Verification items for the finished model (mm, model axes). A direction names the side the tool comes from. Give positions to 0.01 mm unless a question says otherwise; leave off trailing zeros. Loops run counter-clockwise (first coordinate to the right, second up) from the corner with the lowest first, then second, coordinate; pieces in that order, holes last. Notation, with made-up numbers: (69, 28) - (127, 28) arc R32 ccw to (127, 67) - close; hole circle Ø7 at (6, -39). An arc over 180 degrees is marked (long way). One line per question, with ' | ' between items. Start each with the question number.
1. Mould release check, pull along X, two halves, no side actions. Record for faces 5 (the face through (54.27, 10.17, -9.33)), 6 (the face through (6.944, 10.666, -7.841)), 7 (the face through (89.5, 0, 0)): +X half, -X half, draft (parallel to the pull), parting line (faces both ways), or undercut.
2. Depth check by flat-ended pin: pin 1 Ø12 at (y, z) = (-2.5, 8) entering from -X; pin 2 Ø2.5 at (y, z) = (-9.19, -9.19) entering from -X; pin 3 Ø2 at (x, y) = (77.5, -6) entering from -Z; pin 4 Ø4 at (x, z) = (36.5, -2) entering from +Y. Enter the tip coordinate at first touch or a pass-through.
3. Thickness scan on line 1 along X through (y, z) = (6.5, 13); line 2 along Z through (x, y) = (10, 10); line 3 along X through (y, z) = (6.5, 11.5). Record the ranges inside material, lowest first. Write a range as from..to.
4. Tool access check on faces 1 (the face through (2, -9, 0)), 2 (the face through (2, 9, 0)), 3 (the face through (11, 9, -9)), 4 (the face through (73, -4.8, -13.1)). Record the directions out of +Z, -Z, +X, -X, +Y, -Y that give a thin tool (end or side, any length) a straight path to the whole face; none if there is none.
5. Section check C-C, the plane x = 44. Enter the section's corners in (y, z), then the cut area to 3 significant figures.
6. Section check A-A, the plane z = 0. Enter the section's corners in (x, y).
7. Section check B-B, the plane y = 0. Enter the section's corners in (x, z).
8. Section check D-D, the plane x = 26. Enter the section's corners in (y, z).
from build123d import *

# Parameters (mm, degrees)
SKETCH2_W           = 16.5
SKETCH2_H           = 16
SKETCH4_R           = 2
CUT_EXTRUDE1_DEPTH  = 8
SKETCH5_R           = 3
BOSS_EXTRUDE1_DEPTH = 16
CUT_EXTRUDE2_START  = -3
CUT_EXTRUDE2_DEPTH  = 3


with BuildPart() as part:
    # Sketch1 → Revolve1 (revolve)
    with BuildSketch(Plane.XY, mode=Mode.PRIVATE) as revolve1_sk:
        Polygon((0, 0), (0, 10), (3, 10), (3, 16), (35, 16), (35, 13.8), (73, 13.8), (73, 0), align=None)
    revolve(revolve1_sk.sketch.rotate(Axis((0, 0, 0), (1, 0, 0)), 180), axis=Axis((0, 0, 0), (1, 0, 0)))

    # Sketch2 → Revolve2 (revolve)
    with BuildSketch(Plane.XY, mode=Mode.PRIVATE) as revolve2_sk:
        with Locations((81.25, 8)):
            Rectangle(SKETCH2_W, SKETCH2_H)
    revolve(revolve2_sk.sketch.rotate(Axis((73, 0, 0), (1, 0, 0)), 180), axis=Axis((73, 0, 0), (1, 0, 0)))

    # Sketch4 → Cut-Extrude1 (cut)
    with BuildSketch(Plane.ZY.offset(-3)):
        with Locations(Location((9.192388155, 9.192388155, 0), (0, 0, 270))):
            Circle(SKETCH4_R)
        with Locations(Location((9.192388155, -9.192388155, 0), (0, 0, 270))):
            Circle(SKETCH4_R)
        with Locations(Location((-9.192388155, -9.192388155, 0), (0, 0, 270))):
            Circle(SKETCH4_R)
        with Locations(Location((-9.192388155, 9.192388155, 0), (0, 0, 270))):
            Circle(SKETCH4_R)
    extrude(amount=-CUT_EXTRUDE1_DEPTH, mode=Mode.SUBTRACT)

    # Sketch5 → Boss-Extrude1 (add)
    with BuildSketch(Plane.ZY):
        with Locations(Location((0, 0, 0), (0, 0, 270))):
            Circle(SKETCH5_R)
    extrude(amount=BOSS_EXTRUDE1_DEPTH)

    # Sketch6 → Cut-Extrude2 (cut)
    with BuildSketch(Plane.ZY.offset(CUT_EXTRUDE2_START)):
        with BuildLine():
            Line((4.358898944, -9), (-4.358898944, -9))
            ThreePointArc((-4.358898944, -9), (0, -10), (4.358898944, -9))
        make_face()
        with BuildLine():
            ThreePointArc((4.358898944, 9), (0, 10), (-4.358898944, 9))
            Line((-4.358898944, 9), (4.358898944, 9))
        make_face()
    extrude(amount=CUT_EXTRUDE2_DEPTH, mode=Mode.SUBTRACT)


solid = part.part
Results list:
1) face 5: undercut | face 6: draft | face 7: +X half
2) pin 1: x = -16 | pin 2: x = 11 | pin 3: z = -15.2 | pin 4: y = 15.99
3) line 1: 3..35, 73..89.5 | line 2: -12.49..-11.02, -7.36..7.36, 11.02..12.49 | line 3: 3..89.5
4) face 1: +Z, -Z, -X, -Y | face 2: +Z, -Z, -X, +Y | face 3: -X | face 4: none
5) outline: circle Ø27.6 at (0, 0) | area: 598 mm²
6) outline: (-16, -3) - (0, -3) - (0, -9) - (3, -9) - (3, -16) - (35, -16) - (35, -13.8) - (73, -13.8) - (73, -16) - (89.5, -16) - (89.5, 16) - (73, 16) - (73, 13.8) - (35, 13.8) - (35, 16) - (3, 16) - (3, 9) - (0, 9) - (0, 3) - (-16, 3) - close
7) outline: (-16, -3) - (0, -3) - (0, -10) - (3, -10) - (3, -16) - (35, -16) - (35, -13.8) - (73, -13.8) - (73, -16) - (89.5, -16) - (89.5, 16) - (73, 16) - (73, 13.8) - (35, 13.8) - (35, 16) - (3, 16) - (3, 10) - (0, 10) - (0, 3) - (-16, 3) - close
8) outline: circle Ø32 at (0, 0)
